Source: CAD feature listing. Evaluate the final solid. Frame: model axes, mm. Give positions to 0.01 mm unless a question says otherwise; leave off trailing zeros. Write each loop counter-clockwise with the first axis right and the second up, starting at its lowest first coordinate (ties: lowest second). Pieces come first, ordered by that corner, then holes. Notation, with made-up numbers: (64.25, 82) -> (83.25, 82) arc R10 ccw to (83.25, 95) -> close; hole circle Ø2 at (53, -14.75). An arc over 180 degrees is marked (long way). Answer as a JSON object with one key per item and string values. Group by question number.
Item 1: Section query A-A on x = 2.5. Return the cut outline in (y, z).
Item 2: First-contact query: pin 1 Ø3 at (y, z) = (6, 4) entering from +X; pin 2 Ø1 at (x, z) = (4, -2.5) entering from +Y; pin 3 Ø7 at (y, z) = (0, 0) entering from +X. Flat tips, straight axial feed; report the tip coordinate or a pass-through.
Item 3: Ray query, probe 1 along Z at (x, y) = (2.75, 0); probe 2 along Z at (x, y) = (6, -3.5); probe 3 along Z at (x, y) = (6, 6.5). Return the intervals inside material, ascending. Write a range as from..to.
Item 4: Pull-direction query (Z, two-part tool) for faces 1 (the face through (4.227, 2.372, 3.094)), 2 (the face through (8.45, -7.325, -0.161)), 3 (the face through (8.56, 1, -5)); classes: pulls with the +Z half, pulls with the -Z half, needs draft (parallel to the pull), parting line crosses it, or undercut.
Autodesk Inventor part; units mm, degrees
ref_plane "Work Plane1" through (-14.8653, 0, 0) normal (0, -0.866, -0.5) x (1, 0, 0)
ref_plane "YZ Plane" through (0, 0, 0) normal (1, 0, 0) x (0, 1, 0)
ref_plane "XZ Plane" through (0, 0, 0) normal (0, 1, 0) x (-1, 0, 0)
sketch "Sketch1" plane through (0, 0, 0) normal (1, 0, 0) x (0, 1, 0)
  line L0 (-8.2416, 0) -> (-4.1208, 7.1374)
  line L1 (-4.1208, 7.1374) -> (4.1208, 7.1374)
  line L2 (4.1208, 7.1374) -> (8.2416, 0)
  line L3 (8.2416, 0) -> (4.1208, -7.1374)
  line L4 (4.1208, -7.1374) -> (-4.1208, -7.1374)
  line L5 (-4.1208, -7.1374) -> (-8.2416, 0)
  point P0 (0, 0)
  point P1 (0, 0)
  dimension "d0" = 16.4831
extrude "Body" add sketch "Sketch1" along normal blind 8.5598
sketch "Sketch2" plane through (0, 0, 0) normal (0, 0, 1) x (1, 0, 0)
  line L0 (0, 4.1208) -> (0, 8.2416)
  line L1 (0, 8.2416) -> (8.5598, 8.2416)
  line L2 (8.5598, 4.1208) -> (8.5598, 8.2416)
  line L3 (-1.712, 0) -> (10.2718, 0)
  line L4 (0.6375, 8.2416) -> (0, 7.1374)
  line L5 (7.9223, 8.2416) -> (8.5598, 7.1374)
  dimension "d3" = 30
  dimension "d4" = 30
  dimension "d5" = 14.2748
  dimension "d6" = 14.2748
revolve "Chamfer1" cut sketch "Sketch2" angle 360 about axis through (-10, 0, 0) along (1, 0, 0)
sketch "Sketch3" plane through (8.5598, 0, 0) normal (1, 0, 0) x (0, 0, -1)
  arc A0 (-3.5687, -6.1812) -> (3.5687, -6.1812) centre (0, 0) ccw
hole "Thread" at (8.5598, 0, 0) direction (-1, 0, 0) diameter 7.7978 end through all
chamfer "Chamfer2" distance 0.8593 angle 30 1 edges at (8.5598, 0, 3.8989) measured on face at (8.5598, 6.0224, 0.1567)
chamfer "Chamfer3" distance 0.8593 angle 30 1 edges at (0, 0, 3.8989) measured on face at (0, 6.0224, 0.1567)
ref_plane "Work Plane1" through (-14.8653, 0, 0) normal (0, -0.866, -0.5) x (1, 0, 0)
equation "\"d0\" = 1.1547 * SW"
equation "\"d1\" = KOH"
equation "\"d3\" = ANG1"
equation "\"d4\" = ANG2"
equation "\"d5\" = SW0"
equation "\"d6\" = SW01"
equation "\"d8\" = -0.5 * GD1 + 0.5 * NND"
equation "\"d40\" = -0.5 * GD1 + 0.5 * NND"
equation "\"d10\" = -0.5 * GD1 + 0.5 * NND"
equation "\"d41\" = -0.5 * GD1 + 0.5 * NND"
equation "\"ANG1\" = 30deg"
equation "\"ANG2\" = 30deg"
equation "\"NND\" = 9.525"
equation "\"KOH\" = 8.5598"
equation "\"SW\" = 14.2748"
equation "\"SW0\" = SW"
equation "\"SW01\" = SW"
equation "\"THREADDIA\" = 9.525"
equation "\"TOA\" = 30deg"
equation "\"E0\" = 1.155 * SW"
properties part number "AS 2465 - 3/8  UNC" material "Steel, Mild"
Worked answers:
{
 "1": {"outline": "(-8.24, 0) -> (-4.12, -7.14) -> (4.12, -7.14) -> (8.24, 0) -> (4.12, 7.14) -> (-4.12, 7.14) -> close; hole circle Ø7.8 at (0, 0)"},
 "2": {"pin 1": "x = 8.56", "pin 2": "y = 7.09", "pin 3": "through"},
 "3": {"probe 1": "-7.14..-3.9, 3.9..7.14", "probe 2": "-7.14..-1.72, 1.72..7.14", "probe 3": "-3.02..3.02"},
 "4": {"face 1": "undercut", "face 2": "parting line crosses it", "face 3": "needs draft"}
}
